For this review, take the finished solid that the model builds, in its own axes (mm). A direction names the side the tool comes from. Round coordinates to 2 decimals unless told otherwise and drop trailing zeros. Write each loop counter-clockwise with the first axis right and the second up, starting at its lowest first coordinate (ties: lowest second). Pieces come first, ordered by that corner, then holes. Notation, with made-up numbers: (-28, 57) -> (-6, 57) arc R25 cw to (-6, 91) -> close; hole circle Ø5 at (-4.5, 36.5). An arc over 180 degrees is marked (long way). Write each question's results on one line, items separated by ' | '. Start each with the question number.
Item 1: The part is to be moulded in two halves that separate along X. For faces 5 (the cylindrical face through (2.85, 3.23, 21.99)), 6 (the flat face through (18, 6.5, 12)), 7 (the cylindrical face through (181.22, 39.35, 12.35)), say which applies: +X half, -X half, draft (parallel to the pull), parting line (faces both ways), or undercut.
Item 2: Clearance check with flat-ended pins moving along their axes: pin 1 (5 mm diameter, centred on y = 40.5, z = 7, fed in from -X) (3 decimals); pin 2 (10 mm diameter, centred on y = 34, z = 19.5, fed in from +X) (3 decimals); pin 3 (6.5 mm diameter, centred on x = 236.5, z = 9.5, fed in from +Y). State where each tip first meets the part, or that it passes through.
Item 3: Tool access review of faces 1 (the cylindrical face through (54.33, 20.11, 0.57)), 2 (the cylindrical face through (196.796, 20.607, 24.43)), 3 (the flat face through (126, 40, 12)), 4 (the flat face through (234, 6.5, 12)): name each direction out of +Z, -Z, +X, -X, +Y, -Y from which nothing blocks a thin tool from reaching the whole face with its end or side.
Item 4: Add section A-A (x = 229.5). State the section outline as (y, z) points.
Item 5: To check wall thickness, follow line 1 along Y through (x, z) = (107, 4.25); line 2 along X through (y, z) = (17.5, 2.25) (3 decimals); line 3 along X through (y, z) = (26, 14.5) (3 decimals). State the ranges of each line that lie inside material, in increasing order.
from build123d import *

# Parameters (mm, degrees)
F1_DEPTH = 25
F2_R     = 10
F3_R     = 2


with BuildPart() as f1:
    # F0 (on Top) → F1 (new body)
    with BuildSketch(Plane.XY):
        with BuildLine():
            Line((0, 6.5), (0, 0))
            Line((0, 0), (37, 0))
            ThreePointArc((37, 0), (39.683282, 0.633437), (41.8, 2.4))
            Line((41.8, 2.4), (68.2, 37.6))
            ThreePointArc((68.2, 37.6), (70.316718, 39.366563), (73, 40))
            Line((73, 40), (125.75, 40))
            Line((125.75, 40), (125.75, 46.5))
            Line((125.75, 46.5), (68.75, 46.5))
            ThreePointArc((68.75, 46.5), (66.066718, 45.866563), (63.95, 44.1))
            Line((63.95, 44.1), (37.55, 8.9))
            ThreePointArc((37.55, 8.9), (35.433282, 7.133437), (32.75, 6.5))
            Line((32.75, 6.5), (0, 6.5))
        make_face()
    extrude(amount=F1_DEPTH)

    # F2
    f2_edges = [f1.edges().sort_by_distance(p)[0] for p in [
        (0, 3.25, 25),
        (0, 3.25, 0),
    ]]
    fillet(f2_edges, radius=F2_R)

    # F3
    f3_edges = [f1.edges().sort_by_distance(p)[0] for p in [
        (99.375, 40, 25),
        (97.25, 46.5, 25),
    ]]
    fillet(f3_edges, radius=F3_R)

    # F4: F1 across face


with BuildPart() as f1_1:
    add(f1.part)
    add(f1.part.mirror(Plane(origin=(125.75, 43.25, 12.5), x_dir=(0, 1, 0), z_dir=(1, 0, 0))))


solid = f1_1.part
Responses:
1) face 5: -X half | face 6: draft | face 7: undercut
2) pin 1: stops at x = 59.375 | pin 2: stops at x = 198.875 | pin 3: stops at y = 6.5
3) face 1: -Z, -Y | face 2: +Z, -Y | face 3: +Z, -Z, -Y | face 4: +Z, -Z, +X, +Y
4) outline: (0, 2) arc R2 ccw to (2, 0) -> (4.5, 0) arc R2 ccw to (6.5, 2) -> (6.5, 23) arc R2 ccw to (4.5, 25) -> (2, 25) arc R2 ccw to (0, 23) -> close
5) line 1: y = 40 to 46.5 | line 2: x = 44 to 53.125, 198.375 to 207.5 | line 3: x = 50.375 to 59.5, 192 to 201.125
